The figure shows three views and two pictorial views of one solid part (mm, origin at its lowest corner). Answer the questions. Round coordinates to 2 decimals unless told otherwise and drop trailing zeros. Loops run counter-clockwise (first coordinate to the right, second up) from the corner with the lowest first, then second, coordinate; pieces in that order, holes last. Notation, with made-up numbers: (8.5, 26) -> (45.5, 26) arc R17 ccw to (45.5, 39) -> close; hole circle Ø11 at (7.25, 75). An arc over 180 degrees is marked (long way). Write item = value, one per line. Start each with the question number.
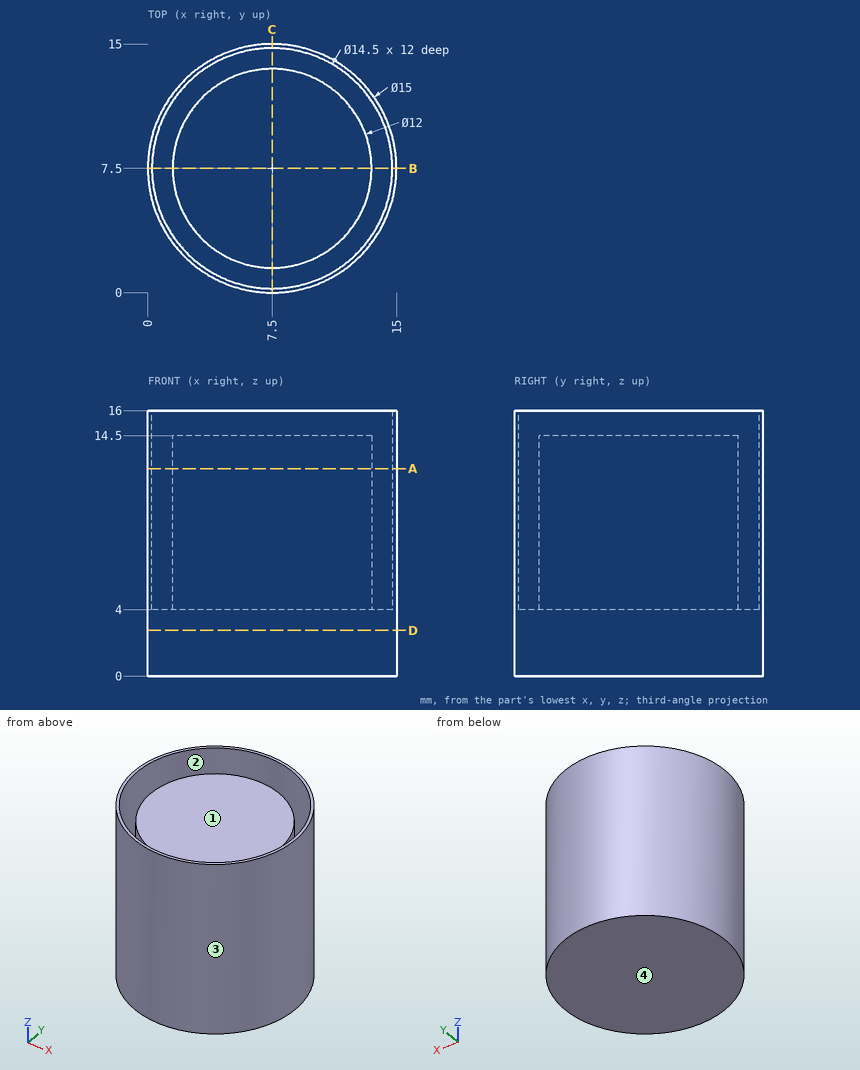
Item 1: Section B-B (y = 7.5) is taken. Determine the outline of the cut face in (x, z), then the cut area to 3 significant figures.
Item 2: Section D-D (z = 2.75) is taken. Determine the outline of the cut face in (x, y).
Item 3: Flat-ended cylindrical pins translate along their axes: pin 1 (5 mm diameter, centred on y = 12.5, z = 8, fed in from -X); pin 2 (1 mm diameter, centred on x = 2.5, z = 3, fed in from +Y); pin 3 (1.5 mm diameter, centred on x = 9, y = 11.5, fed in from +Z); pin 4 (3 mm diameter, centred on x = 13.5, y = 3, fed in from -Z). Find the tip coordinate at first contact, or state that the pin passes through.
Item 4: The mould has two halves that part along X. Classify the marked faces 1, 2, 3 and 4: pulls with the +X half, pulls with the -X half, needs draft (parallel to the pull), parting line crosses it, or undercut.
Item 5: Section A-A (z = 12.5) is taken. Determine the outline of the cut face in (x, y).
Item 6: Find the intervals of material crossed by line 1 along Y through (x, z) = (7.5, 11); line 2 along Y through (x, z) = (3, 7.75); line 3 along Z through (x, y) = (7.75, 14.25), in increasing order. Write a range as [from, to].
Worked answers:
q1.outline = (0, 0) -> (15, 0) -> (15, 16) -> (14.75, 16) -> (14.75, 4) -> (13.5, 4) -> (13.5, 14.5) -> (1.5, 14.5) -> (1.5, 4) -> (0.25, 4) -> (0.25, 16) -> (0, 16) -> close
q1.area = 192 mm2
q2.outline = circle Ø15 at (7.5, 7.5)
q3.pin_1 = 0.43
q3.pin_2 = 13.5
q3.pin_3 = 14.5
q3.pin_4 = 0
q4.face_1 = undercut
q4.face_2 = undercut
q4.face_3 = parting line crosses it
q4.face_4 = needs draft
q5.outline = circle Ø15 at (7.5, 7.5); circle Ø12 at (7.5, 7.5); hole circle Ø14.5 at (7.5, 7.5)
q6.line_1 = [0, 0.25], [1.5, 13.5], [14.75, 15]
q6.line_2 = [1.5, 1.82], [3.53, 11.47], [13.18, 13.5]
q6.line_3 = [0, 4]
